Read the model definition and answer for the solid it produces. Units are mm, in the model's axes. A direction names the side the tool comes from. Give positions to 0.01 mm unless a question says otherwise; leave off trailing zeros. Order: outer loops, then holes, each group sorted by start corner. A loop starts at its lowest first (then second) coordinate and runs counter-clockwise, first axis right, second up.
Item 1: Given pin 1 Ø3 at (y, z) = (3.5, 4) entering from +X; pin 2 Ø1.5 at (x, z) = (-6, 8) entering from +Y; pin 3 Ø5 at (x, z) = (13.5, 1.5) entering from -Y, each flat-ended and moving along its own axis, determine where each tip first touches the part or whether it passes through.
Item 2: A cutting plane is placed at D-D (z = 2.5). Write down the section's boundary in (x, y), plus the area to 3 significant figures.
Item 3: Find the intervals of material crossed by line 1 along Y through (x, z) = (0, 7.25); line 2 along Y through (x, z) = (1, 3.25); line 3 along Z through (x, y) = (5, -3.5), in increasing order.
Item 4: A cutting plane is placed at A-A (z = 6.5). Write down the section's boundary in (x, y), plus the area to 3 significant figures.
Item 5: Which of the six approach directions +Z, -Z, +X, -X, +Y, -Y give full straight-line access (tool end or side, diameter ignored) to faces 1 (the face through (3.47, -15.62, 8.48)), 2 (the face through (-4.006, 1.262, 3.451)), 3 (the face through (-0.65, 1.01, 7.2))?
Item 6: The mould has two halves that part along X. Classify faces 4 (the face through (2.93, -13.18, 3.45)), 5 (the face through (12, -11, 3)), 6 (the face through (3.47, -15.62, 1.48)): +X half, -X half, draft (parallel to the pull), parting line (faces both ways), or undercut.
from build123d import *

# Parameters (mm, degrees)
ESQUISSE1_R                                        = 14.5
BOSS_EXTRU_1_DEPTH                                 = 10
BOSS_EXTRU_2_START                                 = 1
ESQUISSE2_R                                        = 16.5
BOSS_EXTRU_2_DEPTH                                 = 8
ESQUISSE6_R                                        = 13.5
ENL_V_MAT_EXTRU_4_DEPTH                            = 1
CHAMBRAGE_POUR_VIS_T_TE_RONDE_BOMB_E_M_D           = 2.4
CHAMBRAGE_POUR_VIS_T_TE_RONDE_BOMB_E_M_CBORE_D     = 5
CHAMBRAGE_POUR_VIS_T_TE_RONDE_BOMB_E_M_CBORE_DEPTH = 1.6
ESQUISSE13_R                                       = 13.5
ESQUISSE13_R_2                                     = 4.2
ENL_V_MAT_EXTRU_7_DEPTH                            = 7
ENL_V_MAT_EXTRU_8_DEPTH                            = 7
BOSS_EXTRUDE2_START                                = -9
SKETCH2_R                                          = 16.5
SKETCH2_R_2                                        = 14.5
BOSS_EXTRUDE2_DEPTH                                = 10
SKETCH3_R                                          = 22.5
SKETCH3_R_2                                        = 16.5
BOSS_EXTRUDE3_DEPTH                                = 10
FILLET1_R                                          = 1
BOSS_EXTRUDE4_DEPTH                                = 0.5
CIRPATTERN1_COUNT                                  = 70
SKETCH5_R                                          = 40
SKETCH5_R_2                                        = 16
CUT_EXTRUDE1_DEPTH                                 = 20
BOSS_EXTRUDE5_START                                = -3
SKETCH6_R                                          = 18
SKETCH6_R_2                                        = 16
BOSS_EXTRUDE5_DEPTH                                = 4
SKETCH8_R                                          = 13.5
SKETCH8_R_2                                        = 2.5
BOSS_EXTRUDE6_DEPTH                                = 1


with BuildPart() as part:
    # Esquisse1 → Boss.-Extru.1 (new body)
    with BuildSketch(Plane.XY):
        Circle(ESQUISSE1_R)
    extrude(amount=BOSS_EXTRU_1_DEPTH)

    # Esquisse2 → Boss.-Extru.2 (add)
    with BuildSketch(Plane.XY.offset(BOSS_EXTRU_2_START)):
        Circle(ESQUISSE2_R)
    extrude(amount=BOSS_EXTRU_2_DEPTH)

    # Esquisse6 → Enlèv. mat.-Extru.4 (cut)
    with BuildSketch(Plane.XY.offset(10)):
        Circle(ESQUISSE6_R)
    extrude(amount=-ENL_V_MAT_EXTRU_4_DEPTH, mode=Mode.SUBTRACT)

    # Chambrage pour vis à tête ronde bombée M21 (through all)
    with Locations(Plane.XY.offset(9)):
        with Locations((0, 0)):
            CounterBoreHole(CHAMBRAGE_POUR_VIS_T_TE_RONDE_BOMB_E_M_D / 2, CHAMBRAGE_POUR_VIS_T_TE_RONDE_BOMB_E_M_CBORE_D / 2, CHAMBRAGE_POUR_VIS_T_TE_RONDE_BOMB_E_M_CBORE_DEPTH)

    # Esquisse13 → Enlèv. mat.-Extru.7 (cut)
    with BuildSketch(Plane(origin=(0, 0, 0), x_dir=(-1, 0, 0), z_dir=(0, 0, -1))):
        Circle(ESQUISSE13_R)
        Circle(ESQUISSE13_R_2, mode=Mode.SUBTRACT)
    extrude(amount=-ENL_V_MAT_EXTRU_7_DEPTH, mode=Mode.SUBTRACT)

    # Esquisse15 → Enlèv. mat.-Extru.8 (cut)
    with BuildSketch(Plane(origin=(0, 0, 0), x_dir=(-1, 0, 0), z_dir=(0, 0, -1))):
        with BuildLine():
            Line((-2.15, 2.092247595), (-2.15, -2.092247595))
            ThreePointArc((-2.15, -2.092247595), (0, -3), (2.15, -2.092247595))
            Line((2.15, -2.092247595), (2.15, 2.092247595))
            ThreePointArc((2.15, 2.092247595), (0, 3), (-2.15, 2.092247595))
        make_face()
    extrude(amount=-ENL_V_MAT_EXTRU_8_DEPTH, mode=Mode.SUBTRACT)

    # Sketch2 → Boss-Extrude2 (add)
    with BuildSketch(Plane(origin=(0, 0, 1), x_dir=(-1, 0, 0), z_dir=(0, 0, -1)).offset(BOSS_EXTRUDE2_START)):
        Circle(SKETCH2_R)
        Circle(SKETCH2_R_2, mode=Mode.SUBTRACT)
    extrude(amount=BOSS_EXTRUDE2_DEPTH)

    # Sketch3 → Boss-Extrude3 (add)
    with BuildSketch(Plane(origin=(0, 0, 0), x_dir=(-1, 0, 0), z_dir=(0, 0, -1))):
        Circle(SKETCH3_R)
        Circle(SKETCH3_R_2, mode=Mode.SUBTRACT)
    extrude(amount=-BOSS_EXTRUDE3_DEPTH)

    # Fillet1
    fillet1_edges = [part.edges().sort_by_distance(p)[0] for p in [
        (22.5, 0, 10),
        (22.5, 0, 0),
    ]]
    fillet(fillet1_edges, radius=FILLET1_R)

    # Sketch4 → Boss-Extrude4 (add, symmetric)
    with BuildSketch(Plane(origin=(0, 0, 0), x_dir=(0, 0, -1), z_dir=(1, 0, 0))):
        with BuildLine():
            Line((-9, 22.5), (-9, 18))
            Line((-9, 18), (-1, 18))
            Line((-1, 18), (-1, 22.5))
            ThreePointArc((-1, 22.5), (-5, 23.4), (-9, 22.5))
        make_face()
    boss_extrude4 = extrude(amount=BOSS_EXTRUDE4_DEPTH, both=True)

    # CirPattern1: Boss-Extrude4 ×70 about axis
    cirpattern1_axis = Axis((0, 0, 0), (0, 0, 1))
    for i in range(1, CIRPATTERN1_COUNT):
        add(boss_extrude4.rotate(cirpattern1_axis, i * 360 / CIRPATTERN1_COUNT))

    # Sketch5 → Cut-Extrude1 (cut)
    with BuildSketch(Plane(origin=(0, 0, 0), x_dir=(-1, 0, 0), z_dir=(0, 0, -1))):
        Circle(SKETCH5_R)
        Circle(SKETCH5_R_2, mode=Mode.SUBTRACT)
    extrude(amount=-CUT_EXTRUDE1_DEPTH, mode=Mode.SUBTRACT)

    # Sketch6 → Boss-Extrude5 (add)
    with BuildSketch(Plane(origin=(0, 0, 0), x_dir=(-1, 0, 0), z_dir=(0, 0, -1)).offset(BOSS_EXTRUDE5_START)):
        Circle(SKETCH6_R)
        Circle(SKETCH6_R_2, mode=Mode.SUBTRACT)
    extrude(amount=-BOSS_EXTRUDE5_DEPTH)

    # Sketch8 → Boss-Extrude6 (add)
    with BuildSketch(Plane.XY.offset(9)):
        Circle(SKETCH8_R)
        Circle(SKETCH8_R_2, mode=Mode.SUBTRACT)
    extrude(amount=BOSS_EXTRUDE6_DEPTH)


solid = part.part
Response values:
1. pin 1: stops at x = 17.89
1. pin 2: stops at y = 15.11
1. pin 3: stops at y = -13.85
2. outline: circle Ø32 at (0, 0); circle Ø8.4 at (0, 0); hole circle Ø27 at (0, 0); hole (-2.15, -2.09) arc R3 ccw to (2.15, -2.09) - (2.15, 2.09) arc R3 ccw to (-2.15, 2.09) - close
2. area: 264 mm2
3. line 1: y = -16 to -1.2, 1.2 to 16
3. line 2: y = -17.97 to -13.46, -4.08 to -2.83, 2.83 to 4.08, 13.46 to 17.97
3. line 3: z = 7 to 10
4. outline: circle Ø36 at (0, 0); circle Ø8.4 at (0, 0); hole circle Ø27 at (0, 0); hole (-2.15, -2.09) arc R3 ccw to (2.15, -2.09) - (2.15, 2.09) arc R3 ccw to (-2.15, 2.09) - close
4. area: 477 mm2
5. face 1: +Z
5. face 2: -Z
5. face 3: +Z, -Z
6. face 4: undercut
6. face 5: draft
6. face 6: parting line
